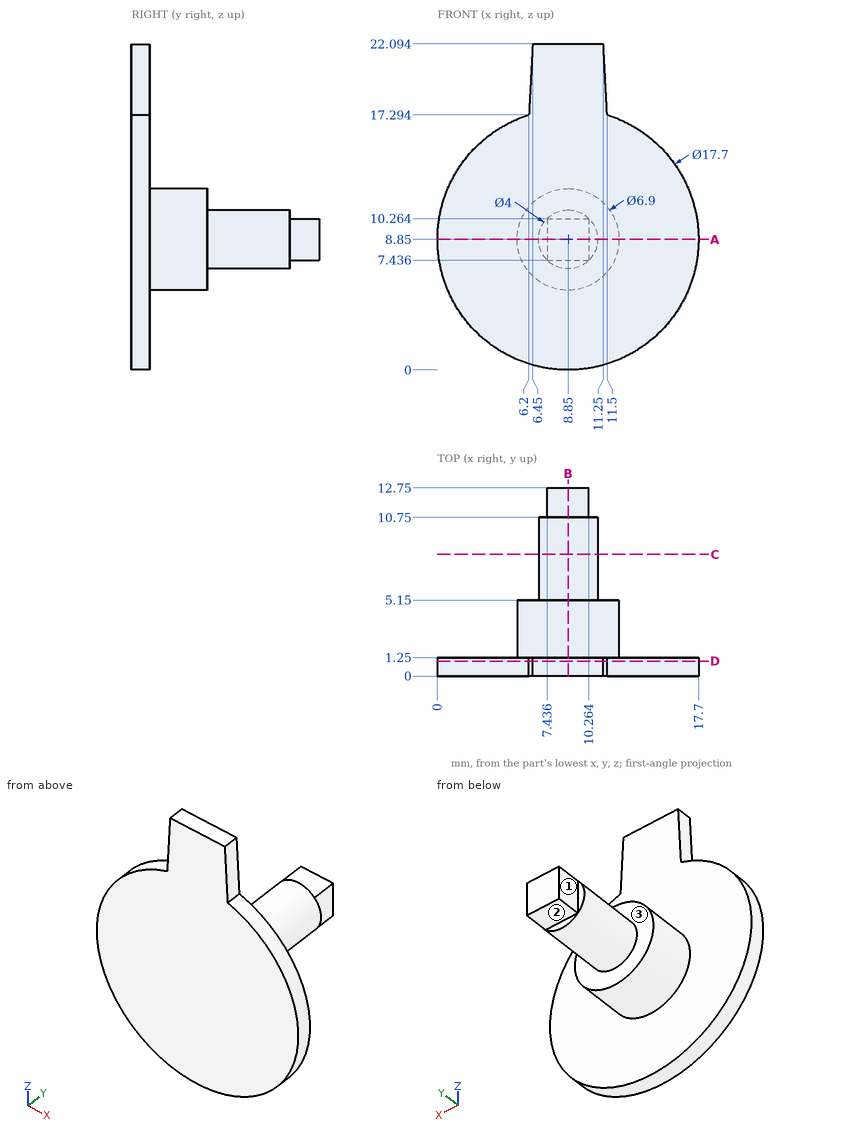
Can you work these out from the drawing? Everything is in mm from the part's minimum corner. A direction names the side the tool comes from. Coordinates: 2 decimals unless noted, no trailing zeros. Order: outer loops, then holes, each group sorted by start corner. A loop starts at its lowest first (then second) coordinate and runs counter-clockwise, first axis right, second up. Notation, with made-up numbers: (-3, 20) -> (12, 20) arc R20 ccw to (12, 26) -> close; hole circle Ø1 at (56.5, -39). An arc over 180 degrees is marked (long way). Use one line per item in the form item = value.
Q1. Imagine slicing it at C-C, the plane y = 8.25. List the corners of the cut face in (x, z) for me.
From the geometry:
outline = circle Ø4 at (8.85, 8.85)
Q2. I need wall thicknesses on L1, parallel to Y at x = 8.5, z = 10.5; L2, parallel to Z at x = 8.5, y = 11.5; L3, parallel to Y at x = 1.25, z = 10.25. Which ranges of each line are inside material? Lowest first, please.
From the geometry:
L1 = 0 to 10.75
L2 = 7.44 to 10.26
L3 = 0 to 1.25
Q3. Imagine slicing it at A-A, the plane z = 8.85. List the corners of the cut face in (x, y) for me, then the cut area to 3 significant figures.
From the geometry:
outline = (0, 0) -> (17.7, 0) -> (17.7, 1.25) -> (12.3, 1.25) -> (12.3, 5.15) -> (10.85, 5.15) -> (10.85, 10.75) -> (10.26, 10.75) -> (10.26, 12.75) -> (7.44, 12.75) -> (7.44, 10.75) -> (6.85, 10.75) -> (6.85, 5.15) -> (5.4, 5.15) -> (5.4, 1.25) -> (0, 1.25) -> close
area = 77.1 mm²
Q4. Will these pins go through, and if not, where does the flat tip stop? P1, Ø0.6, axis at x = 9.5, y = 11.5, coming from the -Z side; P2, Ø1, axis at x = 9, y = 11.5, coming from the +Z side; P3, Ø0.6, axis at y = 11.5, z = 8.5, coming from the -X side.
From the geometry:
P1 = 7.44
P2 = 10.26
P3 = 7.44
Q5. Imagine slicing it at D-D, the plane y = 1. List the corners of the cut face in (x, z) for me, then the cut area to 3 significant figures.
From the geometry:
outline = (6.2, 17.29) arc R8.85 ccw (long way) to (11.5, 17.29) -> (11.25, 22.09) -> (6.45, 22.09) -> close
area = 269 mm²
Q6. Imagine slicing it at B-B, the plane x = 8.85. List the corners of the cut face in (y, z) for me, then the cut area to 3 significant figures.
From the geometry:
outline = (0, 0) -> (1.25, 0) -> (1.25, 5.4) -> (5.15, 5.4) -> (5.15, 6.85) -> (10.75, 6.85) -> (10.75, 7.44) -> (12.75, 7.44) -> (12.75, 10.26) -> (10.75, 10.26) -> (10.75, 10.85) -> (5.15, 10.85) -> (5.15, 12.3) -> (1.25, 12.3) -> (1.25, 22.09) -> (0, 22.09) -> close
area = 82.6 mm²
Q7. Which directions (+Z, -Z, +X, -X, +Y, -Y) give clear straight access to the entire face, cutting with the end or side of a thin tool? Please do the marked faces 1, 2 and 3.
From the geometry:
face_1 = +Z, -Z, -X, +Y
face_2 = -Z, +X, -X, +Y
face_3 = +Y
